from build123d import *

# Parameters (mm, degrees)
SKETCH1_R           = 7.5
SKETCH1_R_2         = 6
BOSS_EXTRUDE1_DEPTH = 15
CHAMFER1_SIZE       = 0.5
SCALE1_SCALE        = 0.317565217


with BuildPart() as part:
    # Sketch1 → Boss-Extrude1 (new body)
    with BuildSketch(Plane.XY):
        Circle(SKETCH1_R)
        Circle(SKETCH1_R_2, mode=Mode.SUBTRACT)
    extrude(amount=BOSS_EXTRUDE1_DEPTH)

    # Chamfer1
    chamfer1_edges = [part.edges().sort_by_distance(p)[0] for p in [
        (-7.5, 0, 15),
    ]]
    chamfer(chamfer1_edges, length=CHAMFER1_SIZE)


with BuildPart() as part_1:
    # Scale1: scaled about (0, 0, 7.455475435)
    add(part.part.scale(SCALE1_SCALE).moved(Location((0, 0, 5.087875758))))


solid = part_1.part
Geometry: final body of the model. Coordinates: model frame, mm. Round coordinates to 2 decimals unless told otherwise and drop trailing zeros. Order: outer loops, then holes, each group sorted by start corner. A loop starts at its lowest first (then second) coordinate and runs counter-clockwise, first axis right, second up.
Q1. Material intervals for probe 1 along Y at (x, z) = (0, 8.85); probe 2 along X at (y, z) = (-0.8, 9.2); probe 3 along X at (y, z) = (-1.15, 8.8), sorted ascending.
Result sheet:
probe 1: y = -2.38 to -1.91, 1.91 to 2.38
probe 2: x = -2.24 to -1.73, 1.73 to 2.24
probe 3: x = -2.09 to -1.52, 1.52 to 2.09
Q2. Section A-A, the plane x = 0. Output: boundary loops of the cut face in (y, z).
Result sheet:
outline: (-2.38, 5.09) - (-1.91, 5.09) - (-1.91, 9.85) - (-2.22, 9.85) - (-2.38, 9.69) - close; (1.91, 5.09) - (2.38, 5.09) - (2.38, 9.69) - (2.22, 9.85) - (1.91, 9.85) - close
Q3. Section C-C, the plane z = 7.1. Output: boundary loops of the cut face in (x, y), and give its area (3 significant figures).
Result sheet:
outline: circle Ø4.76 at (0, 0); hole circle Ø3.81 at (0, 0)
area: 6.42 mm2
Q4. Mould query, pull axis X, two halves, no side actions, for faces 1 (the face through (1.099, -2.113, 7.358)), 2 (the face through (-0.41, -1.86, 7.44)). Classes: released by +X, released by -X, zero draft, split by the parting line, or undercut.
Result sheet:
face 1: split by the parting line
face 2: undercut
